```python
from build123d import *

# Parameters (mm, degrees)
EXTRUDE_2_DEPTH                 = 40
CUT_EXTRUDE_1_DEPTH             = 151.894002532
CUT_EXTRUDE_1_DEPTH_BACK        = 151.894002532
SKETCH_3_R                      = 1.65
EXTRUDE_3_DEPTH                 = 3
MIRROR_2_COPY_1_DEPTH           = 3
CUT_EXTRUDE_2_DEPTH             = 5
SKETCH_10_R                     = 1
CUT_EXTRUDE_3_DEPTH             = 5
EXTRUDE_4_DEPTH                 = 10
CUT_EXTRUDE_4_REACH             = 87.843
CUT_EXTRUDE_4_DIRECTION_2_DEPTH = 7
CUT_EXTRUDE_5_DEPTH             = 91.93404203
CUT_EXTRUDE_5_DEPTH_BACK        = 91.93404203
SKETCH_12_R                     = 1.65


with BuildPart() as part:
    # 草图1 → 凸台-拉伸2 (new body)
    with BuildSketch(Plane.XY):
        Polygon((-75, 0), (75, 0), (75, -12), (70, -12), (70, -5), (-70, -5), (-70, -12), (-75, -12), align=None)
    extrude(amount=EXTRUDE_2_DEPTH)

    # 草图3 → 切除-拉伸1 (cut, two sides: drawn at the far end of the back side and taken through both)
    with BuildSketch(Plane(origin=(-70, 0, 0), x_dir=(0, 0, -1), z_dir=(1, 0, 0)).offset(-CUT_EXTRUDE_1_DEPTH_BACK)):
        with Locations(Location((-10, -9, 0), (0, 0, 90))):
            Circle(SKETCH_3_R)
    extrude(amount=CUT_EXTRUDE_1_DEPTH + CUT_EXTRUDE_1_DEPTH_BACK, mode=Mode.SUBTRACT)

    # 草图4 → 凸台-拉伸3 (add)
    with BuildSketch(Plane(origin=(0, 0, 0), x_dir=(-1, 0, 0), z_dir=(0, 0, -1))):
        Polygon((64, -5), (70, -12), (70, -5), align=None)
    extrude_3 = extrude(amount=-EXTRUDE_3_DEPTH)

    # 镜向1: 凸台-拉伸3 across plane
    add(extrude_3.mirror(Plane.XY.offset(20)))

    # 镜向2: 凸台-拉伸3 across plane
    add(extrude_3.mirror(Plane(origin=(0, 0, 0), x_dir=(0, 0, 1), z_dir=(1, 0, 0))))

    # 镜向2 copy 1 sketch → 镜向2 copy 1 (add)
    with BuildSketch(Plane.XY.offset(40)):
        Polygon((64, -5), (70, -12), (70, -5), align=None)
    extrude(amount=-MIRROR_2_COPY_1_DEPTH)

    # 草图7 → 切除-拉伸2 (cut)
    with BuildSketch(Plane.XZ.offset(5)):
        Polygon((53.2, 22.4), (53.2, 17.6), (53.2, 8), (34, 8), (-37.996196674, 8), (-37.996196674, 32), (34, 32), (53.2, 32), align=None)
    extrude(amount=-CUT_EXTRUDE_2_DEPTH, mode=Mode.SUBTRACT)

    # 草图10 → 切除-拉伸3 (cut)
    with BuildSketch(Plane.XZ.offset(5)):
        with Locations(Location((50, 33.835, 0), (0, 0, 270))):
            Circle(SKETCH_10_R)
        with Locations(Location((40, 33.835, 0), (0, 0, 270))):
            Circle(SKETCH_10_R)
        with Locations(Location((30, 33.835, 0), (0, 0, 270))):
            Circle(SKETCH_10_R)
        with Locations(Location((20, 33.835, 0), (0, 0, 270))):
            Circle(SKETCH_10_R)
        with Locations(Location((10, 33.835, 0), (0, 0, 270))):
            Circle(SKETCH_10_R)
        with Locations(Location((0, 33.835, 0), (0, 0, 270))):
            Circle(SKETCH_10_R)
        with Locations(Location((-10, 33.835, 0), (0, 0, 270))):
            Circle(SKETCH_10_R)
        with Locations(Location((-20, 33.835, 0), (0, 0, 270))):
            Circle(SKETCH_10_R)
        with Locations(Location((50, 6.165, 0), (0, 0, 90))):
            Circle(SKETCH_10_R)
        with Locations(Location((40, 6.165, 0), (0, 0, 90))):
            Circle(SKETCH_10_R)
        with Locations(Location((30, 6.165, 0), (0, 0, 90))):
            Circle(SKETCH_10_R)
        with Locations(Location((20, 6.165, 0), (0, 0, 90))):
            Circle(SKETCH_10_R)
        with Locations(Location((10, 6.165, 0), (0, 0, 90))):
            Circle(SKETCH_10_R)
        with Locations(Location((0, 6.165, 0), (0, 0, 90))):
            Circle(SKETCH_10_R)
        with Locations(Location((-10, 6.165, 0), (0, 0, 90))):
            Circle(SKETCH_10_R)
        with Locations(Location((-20, 6.165, 0), (0, 0, 90))):
            Circle(SKETCH_10_R)
    extrude(amount=-CUT_EXTRUDE_3_DEPTH, mode=Mode.SUBTRACT)

    # 草图11 → 凸台-拉伸4 (add)
    with BuildSketch(Plane.XY.offset(40)):
        Polygon((-75, -12), (-70, -12), (-64, -5), (64, -5), (70, -12), (75, -12), (75, 0), (-75, 0), align=None)
    extrude(amount=EXTRUDE_4_DEPTH)

    # 草图11<3> → 切除-拉伸4 (cut, up to next)
    with BuildSketch(Plane.XY.offset(40), mode=Mode.PRIVATE) as cut_extrude_4_sk1:
        Polygon((-70, -12), (-70, -5), (-64, -5), align=None)
    cut_extrude_4_tool1 = extrude(cut_extrude_4_sk1.sketch, amount=-CUT_EXTRUDE_4_REACH, mode=Mode.PRIVATE) & part.part
    # 草图11<3> → 切除-拉伸4 (cut, up to next)
    with BuildSketch(Plane.XY.offset(40), mode=Mode.PRIVATE) as cut_extrude_4_sk2:
        Polygon((64, -5), (70, -5), (70, -12), align=None)
    cut_extrude_4_tool2 = extrude(cut_extrude_4_sk2.sketch, amount=-CUT_EXTRUDE_4_REACH, mode=Mode.PRIVATE) & part.part
    add(cut_extrude_4_tool1.solids().sort_by_distance((-68, -7.333333, 40))[0], mode=Mode.SUBTRACT)
    add(cut_extrude_4_tool2.solids().sort_by_distance((68, -7.333333, 40))[0], mode=Mode.SUBTRACT)

    # 草图11<3> → 切除-拉伸4 direction 2 (cut)
    with BuildSketch(Plane.XY.offset(40)):
        Polygon((-70, -12), (-70, -5), (-64, -5), align=None)
        Polygon((64, -5), (70, -5), (70, -12), align=None)
    extrude(amount=CUT_EXTRUDE_4_DIRECTION_2_DEPTH, mode=Mode.SUBTRACT)

    # 草图12 → 切除-拉伸5 (cut, two sides: drawn at the far end of the back side and taken through both)
    with BuildSketch(Plane(origin=(0, 0, 0), x_dir=(0, 0, -1), z_dir=(1, 0, 0)).offset(-CUT_EXTRUDE_5_DEPTH_BACK)):
        with Locations((-40, -9)):
            Circle(SKETCH_12_R)
    extrude(amount=CUT_EXTRUDE_5_DEPTH + CUT_EXTRUDE_5_DEPTH_BACK, mode=Mode.SUBTRACT)


solid = part.part
```
Source: CAD feature listing. Evaluate the final solid. Frame: model axes, mm. A direction names the side the tool comes from. Round coordinates to 2 decimals unless told otherwise and drop trailing zeros. Loops run counter-clockwise (first coordinate to the right, second up) from the corner with the lowest first, then second, coordinate; pieces in that order, holes last.
1. Ray query, L1, parallel to Z at x = 73.8, y = -9; L2, parallel to X at y = -1.25, z = 14; L3, parallel to X at y = -6.5, z = 12.5. Return the intervals inside material, ascending.
2. Mould query, pull axis Y, two halves, no side actions, for faces 1 (the cylindrical face through (-72.54, -10.31, 9)), 2 (the flat face through (1, 0, 36)), 3 (the flat face through (-73, -12, 25)), 4 (the flat face through (-1, -3, 0)). Classes: released by +Y, released by -Y, zero draft, split by the parting line, or undercut.
3. Section query D-D on y = -3.25. Give the number of separate pieces and of enclosed holes in the cut face, and give its area (3 significant figures).
4. Section query C-C on z = 18. Output: boundary loops of the cut face in (x, y), and give its area (3 significant figures).
5. Contact query for flat-ended pins moving along their axis: pin 1 (2.5 mm diameter, centred on x = -10, z = 6.165, fed in from -Y); pin 2 (1.8 mm diameter, centred on x = 40, z = 6.165, fed in from +Y). Output: stop coordinate, or through.
6. Access query for faces 5 (the flat face through (67, -8.5, 1.5)), 6 (the flat face through (-68, -7, 47)), 7 (the flat face through (-37.996, -3, 20)). Directions: +Z, -Z, +X, -X, +Y, -Y. A direction counts if a zero-diameter tool reaches every point of the face in a straight line with its end or side. Return the directions, or none.
7. Section query B-B on x = -30. Output: boundary loops of the cut face in (y, z), and give its area (3 significant figures).
8. Section query A-A on z = 40. Output: boundary loops of the cut face in (x, y).
Answers below:
1. L1: z = 0 to 8.35, 11.65 to 38.35, 41.65 to 50
1. L2: x = -75 to -38, 53.2 to 75
1. L3: x = -75 to -70, 70 to 75
2. face 1: undercut
2. face 2: released by +Y
2. face 3: released by -Y
2. face 4: zero draft
3. separate pieces: 1
3. enclosed holes: 17
3. area: 5,260 mm2
4. outline: (-75, -12) - (-70, -12) - (-70, -5) - (-38, -5) - (-38, 0) - (-75, 0) - close; (53.2, -5) - (70, -5) - (70, -12) - (75, -12) - (75, 0) - (53.2, 0) - close
4. area: 364 mm2
5. pin 1: stops at y = -5
5. pin 2: passes through
6. face 5: +Z, -Z, -Y
6. face 6: -Y
6. face 7: +Y, -Y
7. outline: (-5, 0) - (0, 0) - (0, 8) - (-5, 8) - close; (-5, 32) - (0, 32) - (0, 50) - (-5, 50) - close
7. area: 130 mm2
8. outline: (-75, -12) - (-70, -12) - (-70, -10.65) - (-75, -10.65) - close; (-75, -7.35) - (-70, -7.35) - (-70, -5) - (70, -5) - (70, -7.35) - (75, -7.35) - (75, 0) - (-75, 0) - close; (70, -12) - (75, -12) - (75, -10.65) - (70, -10.65) - close
